```python
from build123d import *

# Parameters (mm, degrees)
SKETCH2_R           = 2.5
SKETCH2_W           = 2.05
SKETCH2_H           = 1.3
BOSS_EXTRUDE1_DEPTH = 10
FILLET1_R           = 1
SKETCH3_W           = 2.05
SKETCH3_H           = 1.3
BOSS_EXTRUDE5_DEPTH = 16
SKETCH4_R           = 10
THUMB_STICK_DEPTH   = 3.5
FILLET2_R           = 1
FILLET3_R           = 1
SKETCH4_4_R         = 8.9
CUT_EXTRUDE1_DEPTH  = 1
FILLET5_R           = 0.1


with BuildPart() as part:
    # Sketch2 → Boss-Extrude1 (new, symmetric)
    with BuildSketch(Plane(origin=(0, 0, 0), x_dir=(1, 0, 0), z_dir=(0, 1, 0))):
        with Locations(Location((0, 0, 0), (0, 0, 270))):
            Circle(SKETCH2_R)
        Rectangle(SKETCH2_W, SKETCH2_H, mode=Mode.SUBTRACT)
    extrude(amount=BOSS_EXTRUDE1_DEPTH, both=True)

    # Fillet1
    fillet1_edges = [part.edges().sort_by_distance(p)[0] for p in [
        (0, 10, -2.5),
    ]]
    fillet(fillet1_edges, radius=FILLET1_R)

    # Sketch3 → Boss-Extrude5 (add)
    with BuildSketch(Plane(origin=(0, 10, 0), x_dir=(1, 0, 0), z_dir=(0, 1, 0))):
        Rectangle(SKETCH3_W, SKETCH3_H)
    extrude(amount=-BOSS_EXTRUDE5_DEPTH)

    # Sketch4 → Thumb Stick (add)
    with BuildSketch(Plane(origin=(0, 10, 0), x_dir=(1, 0, 0), z_dir=(0, 1, 0))):
        with Locations(Location((0, 0, 0), (0, 0, 270))):
            Circle(SKETCH4_R)
    extrude(amount=-THUMB_STICK_DEPTH)

    # Fillet2
    fillet2_edges = [part.edges().sort_by_distance(p)[0] for p in [
        (0, 6.5, -10),
    ]]
    fillet(fillet2_edges, radius=FILLET2_R)

    # Fillet3
    fillet3_edges = [part.edges().sort_by_distance(p)[0] for p in [
        (0, 10, -10),
    ]]
    fillet(fillet3_edges, radius=FILLET3_R)

    # Sketch4<4> → Cut-Extrude1 (cut)
    with BuildSketch(Plane(origin=(0, 10, 0), x_dir=(1, 0, 0), z_dir=(0, 1, 0))):
        with Locations(Location((0, 0, 0), (0, 0, 270))):
            Circle(SKETCH4_4_R)
    extrude(amount=-CUT_EXTRUDE1_DEPTH, mode=Mode.SUBTRACT)

    # Fillet5
    fillet5_edges = [part.edges().sort_by_distance(p)[0] for p in [
        (0, 10, -8.9),
    ]]
    fillet(fillet5_edges, radius=FILLET5_R - 0.0001)  # a hair under: the kernel refuses the full size


solid = part.part
```
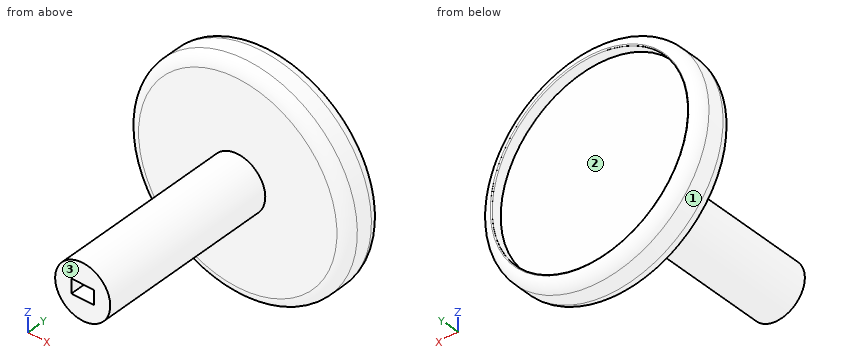
Verification items for the finished model (mm, model axes). Face numbers are marked on the shaded views. Round coordinates to 2 decimals unless told otherwise and drop trailing zeros. Write each loop counter-clockwise with the first axis right and the second up, starting at its lowest first coordinate (ties: lowest second). Pieces come first, ordered by that corner, then holes. Notation, with made-up numbers: (-37, -27.75) -> (14, -27.75) arc R21 cw to (14, -23.75) -> close; hole circle Ø11 at (44.5, 68.5). An arc over 180 degrees is marked (long way). Write each question's results on one line, items separated by ' | '. Start each with the question number.
1. Draft check along X on the marked faces 1, 2 and 3. Enter one of: +X half, -X half, draft (parallel to the pull), parting line (faces both ways), or undercut.
2. Depth check by flat-ended pin: P1, Ø3, axis at x = 5.5, z = 2.5, coming from the -Y side; P2, Ø10, axis at x = 4, y = -6, coming from the -Z side; P3, Ø1.5, axis at y = 5.5, z = 5, coming from the +X side; P4, Ø1, axis at y = -0.5, z = -2, coming from the -X side. Enter the tip coordinate at first touch or a pass-through.
3. Cross-section at C-C (y = -3.5). Enter the section's corners in (x, z), then the cut area to 3 significant figures.
4. Material ranges on probe 1 along Y at (x, z) = (-3.25, -5.25); probe 2 along X at (y, z) = (9.6, 0); probe 3 along X at (y, z) = (9.3, 0), recorded low to high. Write a range as from..to.
Solutions:
1) face 1: parting line | face 2: undercut | face 3: draft
2) P1: stops at y = 6.5 | P2: stops at z = -2.5 | P3: passes through | P4: stops at x = -2
3) outline: circle Ø5 at (0, 0) | area: 19.6 mm2
4) probe 1: y = 6.5..9 | probe 2: x = -9.8..-8.9, 8.9..9.8 | probe 3: x = -9.95..-8.9, 8.9..9.95
